Autodesk Inventor part; units mm, degrees
ref_plane "Work Plane3" through (16, 10, 0) normal (-1, 0, 0) x (0, -1, 0)
ref_plane "YZ Plane" through (0, 0, 0) normal (1, 0, 0) x (0, 1, 0)
ref_plane "XZ Plane" through (0, 0, 0) normal (0, 1, 0) x (-1, 0, 0)
sketch "Sketch1" plane through (0, 0, 0) normal (0, 0, 1) x (1, 0, 0)
  arc A0 (3.8592, 10.1235) -> (3.8, 10.125) centre (3.8, 8.925) ccw construction
  line L0 (1.2, 10.125) -> (3.8, 10.125) construction
  arc A1 (1.2, 10.125) -> (0, 8.925) centre (1.2, 8.925) ccw construction
  line L1 (0, 6) -> (0, 8.925) construction
  arc A2 (0, 6) -> (0, -6) centre (0, 0) ccw
  line L2 (0, -8.925) -> (0, -6) construction
  arc A3 (0, -8.925) -> (1.2, -10.125) centre (1.2, -8.925) ccw construction
  line L3 (1.2, -10.125) -> (3.8, -10.125) construction
  arc A4 (3.8, -10.125) -> (3.8592, -10.1235) centre (3.8, -8.925) ccw construction
  line L4 (3.8592, 10.1235) -> (3.8592, -10.1235) construction
  circle A5 centre (1, 0) radius 2
  arc A6 (28.2, 10.125) -> (28.1408, 10.1235) centre (28.2, 8.925) ccw
  line L5 (28.1408, -10.1235) -> (28.1408, 10.1235)
  arc A7 (28.1408, -10.1235) -> (28.2, -10.125) centre (28.2, -8.925) ccw
  line L6 (28.2, -10.125) -> (30.8, -10.125)
  arc A8 (30.8, -10.125) -> (32, -8.925) centre (30.8, -8.925) ccw
  line L7 (32, -8.925) -> (32, -6)
  arc A9 (32, -6) -> (32, 6) centre (32, 0) ccw
  line L8 (32, 6) -> (32, 8.925)
  arc A10 (32, 8.925) -> (30.8, 10.125) centre (30.8, 8.925) ccw
  line L9 (28.2, 10.125) -> (30.8, 10.125)
  circle A11 centre (31, 0) radius 2
  line L10 (5.0533, -8.925) -> (5.0533, 8.925) construction
  line L11 (26.9467, 8.925) -> (26.9467, -8.925)
  line L12 (0, -6) -> (3.8592, -6)
  line L13 (0, 6) -> (3.8592, 6)
  line L14 (3.8592, -6) -> (3.8592, 6)
  point P0 (25.5, -25.375)
sketch "Sketch2" plane through (0, 0, 0) normal (0, 1, 0) x (-1, 0, 0)
  arc A0 (-26.9467, 0) -> (-5.0533, 0) centre (-16, 0) ccw
  arc A1 (-32, 0) -> (0, 0) centre (-16, 0) ccw
  line L0 (-28.1408, 0) -> (-26.9467, 0)
  line L1 (-5.0533, 0) -> (-3.8592, 0)
  line L2 (0, 0) -> (-5.0533, 0)
  line L3 (-26.9467, 0) -> (-32, 0)
  point P0 (-26.9467, 0)
extrude "Extrusion1" add sketch "Sketch2" along normal mid plane 20
extrude "Extrusion2" add sketch "Sketch1" against normal blind 13 contours L13 L14 L12 A2
sketch "Sketch3" plane through (3.8592, -6, -10.4211) normal (1, 0, 0) x (0, 0, -1)
  line L0 (0, 0) -> (0, 12)
  line L1 (0, 0) -> (2.5789, 0)
  line L2 (2.5789, 0) -> (2.5789, 12)
  line L3 (0, 12) -> (2.5789, 12)
  point P0 (-10.4211, 6)
extrude "Extrusion3" add sketch "Sketch3" along normal blind 5
ref_plane "Work Plane3" through (16, 10, 0) normal (-1, 0, 0) x (0, -1, 0)
ref_plane "Work Plane1" through (0, 10, 0) normal (-1, 0, 0) x (0, -1, 0)
ref_plane "Work Plane2" through (32, 10, 0) normal (-1, 0, 0) x (0, -1, 0)
mirror "Mirror1" about plane through (16, 10, 0) normal (-1, 0, 0) of "Extrusion3", "Extrusion2"
extrude "Extrusion4" cut sketch "Sketch1" against normal through all contours A5
mirror "Mirror2" about plane through (16, 10, 0) normal (-1, 0, 0) of "Extrusion4"
fillet "Fillet1" radius 2 8 edges at (3.3363, -6, -13) (3.3363, 6, -13) (-6, 0, -13) (28.6637, -6, -13) (28.6637, 6, -13) (38, 0, -13) (16, 10, -16) (16, -10, -16)
properties part number "Abrazadera"
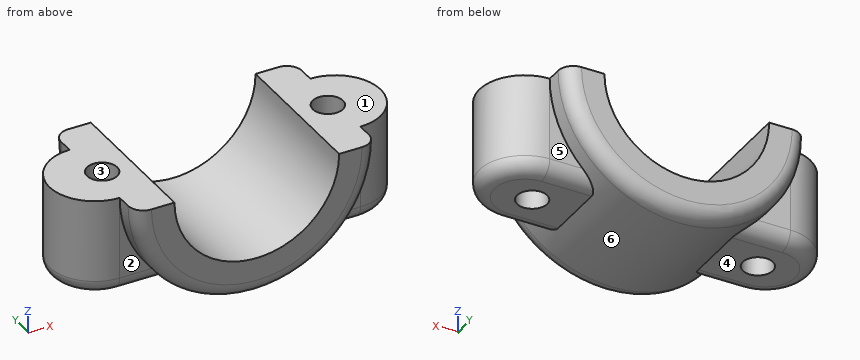
Geometry check sheet. Reference: the model listing, model coordinates, mm. Face numbers are marked on the shaded views. A direction names the side the tool comes from. Round coordinates to 2 decimals unless told otherwise and drop trailing zeros. Loops run counter-clockwise (first coordinate to the right, second up) from the corner with the lowest first, then second, coordinate; pieces in that order, holes last. Notation, with made-up numbers: (2.5, -15) -> (9.5, -15) arc R16 ccw to (9.5, -10) -> close; hole circle Ø9 at (-1.75, 46). An arc over 180 degrees is marked (long way). Use a Markdown table: item, result.
(1) Scan lines: probe 1 along Y at (x, z) = (31, -9.75); probe 2 along X at (y, z) = (0, -5.75); probe 3 along X at (y, z) = (0, -7). Record each from-to range of solid material in increasing order.
Calculated:
| item | result |
|---|---|
| probe 1 | -6 to -2, 2 to 6 |
| probe 2 | -6 to -1, 3 to 6.69, 25.31 to 29, 33 to 38 |
| probe 3 | -6 to -1, 3 to 7.58, 24.42 to 29, 33 to 38 |
(2) Sectioned sample at B-B (y = -7.5). Enter the section's corners in (x, z), then the cut area to 3 significant figures.
Calculated:
| item | result |
|---|---|
| outline | (0, 0) arc R16 ccw to (32, 0) -> (26.95, 0) arc R10.95 cw to (5.05, 0) -> close |
| area | 214 mm² |
(3) Set-up check for the marked faces 4, 5 and 6: record each of +Z, -Z, +X, -X, +Y, -Y from which the full face is reachable in a straight line by a thin tool's end or side.
Calculated:
| item | result |
|---|---|
| face 4 | -Z, -X, +Y, -Y |
| face 5 | -Z, +X, +Y |
| face 6 | -Z |
(4) Go/stop test with flat-tipped pins: P1, Ø2, axis at x = -1, z = -2, coming from the +Y side; P2, Ø5, axis at y = 5, z = -2, coming from the +X side; P3, Ø6.5, axis at x = 1, y = 0, coming from the -Z side. Record where each tip stops, or that it passes through.
Calculated:
| item | result |
|---|---|
| P1 | y = 6 |
| P2 | x = 37.45 |
| P3 | z = -13 |
(5) Sectioned sample at A-A (z = -5.25). Give the number of separate pieces and of enclosed holes in the cut face, then the cut area to 3 significant figures.
Calculated:
| item | result |
|---|---|
| separate pieces | 2 |
| enclosed holes | 2 |
| area | 326 mm² |
(6) Mould release check, pull along Y, two halves, no side actions. Record for the marked faces 1, 2 and 3: released by +Y, released by -Y, zero draft, split by the parting line, or undercut.
Calculated:
| item | result |
|---|---|
| face 1 | zero draft |
| face 2 | released by -Y |
| face 3 | undercut |
(7) Sectioned sample at C-C (x = 16). Enter the section's corners in (y, z), then the cut area to 3 significant figures.
Calculated:
| item | result |
|---|---|
| outline | (-10, -14) arc R2 ccw to (-8, -16) -> (8, -16) arc R2 ccw to (10, -14) -> (10, -10.95) -> (-10, -10.95) -> close |
| area | 99.3 mm² |
